```python
from build123d import *

# Parameters (mm, degrees)
BOSS_EXTRUDE1_DEPTH   = 12.7
FILLET1_R             = 1.27
F_6_32_TAPPED_HOLE1_D = 2.7051
F_6_32_TAPPED_HOLE2_D = 2.7051


with BuildPart() as part:
    # Sketch1 → Boss-Extrude1 (new body)
    with BuildSketch(Plane.XY):
        Polygon((0, 0), (14.2748, 0), (14.2748, 14.2748), (12.7, 14.2748), (12.7, 1.5748), (0, 1.5748), align=None)
    extrude(amount=BOSS_EXTRUDE1_DEPTH)

    # Fillet1
    fillet1_edges = [part.edges().sort_by_distance(p)[0] for p in [
        (12.7, 1.5748, 6.35),
        (14.2748, 0, 6.35),
    ]]
    fillet(fillet1_edges, radius=FILLET1_R)

    # #6-32 Tapped Hole1 (through all)
    with Locations(Plane.ZY.offset(-12.7)):
        with Locations((6.35, 10.4648)):
            Hole(F_6_32_TAPPED_HOLE1_D / 2)

    # #6-32 Tapped Hole2 (through all)
    with Locations(Plane(origin=(0, 1.5748, 0), x_dir=(1, 0, 0), z_dir=(0, 1, 0))):
        with Locations((3.81, -6.35)):
            Hole(F_6_32_TAPPED_HOLE2_D / 2)


solid = part.part
```
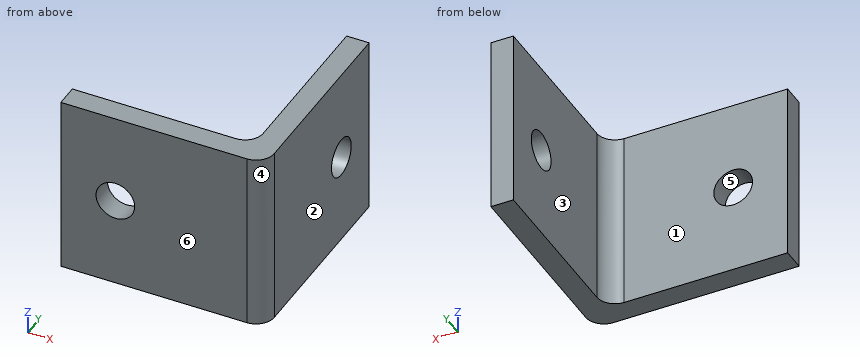
Geometry check sheet. Reference: the model listing, model coordinates, mm. Face numbers are marked on the shaded views. A direction names the side the tool comes from. Round coordinates to 2 decimals unless told otherwise and drop trailing zeros. Order: outer loops, then holes, each group sorted by start corner. A loop starts at its lowest first (then second) coordinate and runs counter-clockwise, first axis right, second up. Notation, with made-up numbers: (86.25, 61.5) -> (110.25, 61.5) arc R22 ccw to (110.25, 77.5) -> close; hole circle Ø11 at (3.25, 62.25). An arc over 180 degrees is marked (long way). Return JSON: item names as keys, results as strings. Group by question number.
Q1. Section check C-C, the plane z = 2.5. Record the boundary of the cut face in (x, y), plus the area to 3 significant figures.
Q2. Section check B-B, the plane z = 6.35. Record the boundary of the cut face in (x, y).
Q3. Release check for a two-part mould opening along X. For the marked faces 3, 4, 5 and 6 record: released by +X, released by -X, zero draft, split by the parting line, or undercut.
Q4. Section check A-A, the plane x = 3.81. Record the boundary of the cut face in (y, z), plus the area to 3 significant figures.
Q5. Section check D-D, the plane x = 8. Record the boundary of the cut face in (y, z), plus the area to 3 significant figures.
Q6. Gauge pin test, flat end, axial feed: pin 1 (5.5 mm diameter, centred on y = 7.5, z = 7, fed in from -X). Record the tip position at first contact, or that the pin passes through.
Q7. Material ranges on probe 1 along X at (y, z) = (1.25, 6.35); probe 2 along Z at (x, y) = (3.81, 0.55); probe 3 along Y at (x, z) = (2, 11), recorded low to high. Write a range as from..to.
Q8. Tool access check on the marked faces 1 and 2. Record the directions out of +Z, -Z, +X, -X, +Y, -Y that give a thin tool (end or side, any length) a straight path to the whole face; none if there is none.
Numbers:
{
 "1": {"outline": "(0, 0) -> (13, 0) arc R1.27 ccw to (14.27, 1.27) -> (14.27, 14.27) -> (12.7, 14.27) -> (12.7, 2.84) arc R1.27 cw to (11.43, 1.57) -> (0, 1.57) -> close", "area": "42.5 mm^2"},
 "2": {"outline": "(0, 0) -> (2.46, 0) -> (2.46, 1.57) -> (0, 1.57) -> close; (5.16, 0) -> (13, 0) arc R1.27 ccw to (14.27, 1.27) -> (14.27, 9.11) -> (12.7, 9.11) -> (12.7, 2.84) arc R1.27 cw to (11.43, 1.57) -> (5.16, 1.57) -> close; (12.7, 11.82) -> (14.27, 11.82) -> (14.27, 14.27) -> (12.7, 14.27) -> close"},
 "3": {"face 3": "released by -X", "face 4": "released by +X", "face 5": "undercut", "face 6": "zero draft"},
 "4": {"outline": "(0, 0) -> (1.57, 0) -> (1.57, 5) -> (0, 5) -> close; (0, 7.7) -> (1.57, 7.7) -> (1.57, 12.7) -> (0, 12.7) -> close", "area": "15.7 mm^2"},
 "5": {"outline": "(0, 0) -> (1.57, 0) -> (1.57, 12.7) -> (0, 12.7) -> close", "area": "20.0 mm^2"},
 "6": {"pin 1": "x = 12.7"},
 "7": {"probe 1": "0..2.46, 5.16..14.27", "probe 2": "0..5, 7.7..12.7", "probe 3": "0..1.57"},
 "8": {"face 1": "+Z, -Z, -X, +Y", "face 2": "+Z, -Z, +X, +Y, -Y"}
}
